```python
from build123d import *

# Parameters (mm, degrees)
SKETCH1_W                                      = 137.49
SKETCH1_H                                      = 96.345
SKETCH1_R                                      = 2.5
SKETCH1_W_2                                    = 10.25
SKETCH1_H_2                                    = 3.4925
BOSS_EXTRUDE1_DEPTH                            = 3.175
CUT_EXTRUDE1_START                             = -1
SKETCH1_3_W                                    = 10.25
SKETCH1_3_H                                    = 3.4925
CUT_EXTRUDE1_DEPTH                             = 5.175
M2_5_CLEARANCE_HOLE1_D                         = 2.9
M2_5_CLEARANCE_HOLE1_CSINK_D                   = 2.95
M2_5_CLEARANCE_HOLE1_CSINK_ANGLE               = 100
MIRROR1_START                                  = -1
MIRROR1_AT_THE_SECOND_PLANE_COPY_1_SKETC_W     = 10.25
MIRROR1_AT_THE_SECOND_PLANE_COPY_1_SKETC_H     = 3.4925
MIRROR1_AT_THE_SECOND_PLANE_COPY_1_DEPTH       = 5.175
MIRROR1_AT_THE_SECOND_PLANE_COPY_2_D           = 2.9
MIRROR1_AT_THE_SECOND_PLANE_COPY_2_CSINK_D     = 2.95
MIRROR1_AT_THE_SECOND_PLANE_COPY_2_CSINK_ANGLE = 100
SKETCH4_W                                      = 82.49
SKETCH4_H                                      = 14
CUT_EXTRUDE2_DEPTH                             = 1
CUT_EXTRUDE2_DEPTH_BACK                        = 4.175
FILLET1_R                                      = 1.5
FILLET2_R                                      = 1
M2_5_CLEARANCE_HOLE2_D                         = 2.9


with BuildPart() as part:
    # Sketch1 → Boss-Extrude1 (new body)
    with BuildSketch(Plane(origin=(0, 0, 0), x_dir=(1, 0, 0), z_dir=(0, 1, 0))):
        Rectangle(SKETCH1_W, SKETCH1_H)
        with Locations((-49.57, 44.1725)):
            Circle(SKETCH1_R, mode=Mode.SUBTRACT)
        with Locations((-58.57, 44.1725)):
            Rectangle(SKETCH1_W_2, SKETCH1_H_2, mode=Mode.SUBTRACT)
        with Locations((-58.57, 44.1725)):
            Rectangle(SKETCH1_W_2, SKETCH1_H_2)
        with Locations((-49.57, 44.1725)):
            Circle(SKETCH1_R)
    extrude(amount=BOSS_EXTRUDE1_DEPTH)

    # Sketch1<3> → Cut-Extrude1 (cut)
    with BuildSketch(Plane(origin=(0, 0, 0), x_dir=(1, 0, 0), z_dir=(0, 1, 0)).offset(CUT_EXTRUDE1_START)):
        with Locations((-58.57, 44.1725)):
            Rectangle(SKETCH1_3_W, SKETCH1_3_H)
    cut_extrude1 = extrude(amount=CUT_EXTRUDE1_DEPTH, mode=Mode.SUBTRACT)

    # M2.5 Clearance Hole1 (through all)
    with Locations(Plane(origin=(0, 3.175, 0), x_dir=(1, 0, 0), z_dir=(0, 1, 0))):
        with Locations((-49.57, 44.1725)):
            m2_5_clearance_hole1 = CounterSinkHole(M2_5_CLEARANCE_HOLE1_D / 2, M2_5_CLEARANCE_HOLE1_CSINK_D / 2, counter_sink_angle=M2_5_CLEARANCE_HOLE1_CSINK_ANGLE)

    # Mirror1: Cut-Extrude1, M2.5 Clearance Hole1 across plane
    add(cut_extrude1.mirror(Plane(origin=(0, 0, 0), x_dir=(0, 0, 1), z_dir=(1, 0, 0))), mode=Mode.SUBTRACT)
    add(m2_5_clearance_hole1.mirror(Plane(origin=(0, 0, 0), x_dir=(0, 0, 1), z_dir=(1, 0, 0))), mode=Mode.SUBTRACT)

    # Mirror1 at the second plane: M2.5 Clearance Hole1, Cut-Extrude1 across plane
    add(m2_5_clearance_hole1.mirror(Plane.XY), mode=Mode.SUBTRACT)
    add(cut_extrude1.mirror(Plane.XY), mode=Mode.SUBTRACT)

    # Mirror1 at the second plane copy 1 sketc → Mirror1 at the second plane copy 1 (cut)
    with BuildSketch(Plane(origin=(0, 0, 0), x_dir=(-1, 0, 0), z_dir=(0, 1, 0)).offset(MIRROR1_START)):
        with Locations((-58.57, 44.1725)):
            Rectangle(MIRROR1_AT_THE_SECOND_PLANE_COPY_1_SKETC_W, MIRROR1_AT_THE_SECOND_PLANE_COPY_1_SKETC_H)
    extrude(amount=MIRROR1_AT_THE_SECOND_PLANE_COPY_1_DEPTH, mode=Mode.SUBTRACT)

    # Mirror1 at the second plane copy 2 (through all)
    with Locations(Plane(origin=(0, 3.175, 0), x_dir=(-1, 0, 0), z_dir=(0, 1, 0))):
        with Locations((-49.57, 44.1725)):
            CounterSinkHole(MIRROR1_AT_THE_SECOND_PLANE_COPY_2_D / 2, MIRROR1_AT_THE_SECOND_PLANE_COPY_2_CSINK_D / 2, counter_sink_angle=MIRROR1_AT_THE_SECOND_PLANE_COPY_2_CSINK_ANGLE)

    # Sketch4 → Cut-Extrude2 (cut, two sides)
    with BuildSketch(Plane(origin=(0, 3.175, 0), x_dir=(1, 0, 0), z_dir=(0, 1, 0))) as cut_extrude2_sk:
        with Locations((19.5, 30.1725)):
            Rectangle(SKETCH4_W, SKETCH4_H)
    extrude(amount=CUT_EXTRUDE2_DEPTH, mode=Mode.SUBTRACT)
    extrude(cut_extrude2_sk.sketch, amount=-CUT_EXTRUDE2_DEPTH_BACK, mode=Mode.SUBTRACT)

    # Fillet1
    fillet1_edges = [part.edges().sort_by_distance(p)[0] for p in [
        (-21.745, 1.5875, -23.1725),
        (-21.745, 1.5875, -37.1725),
        (60.745, 1.5875, -37.1725),
        (60.745, 1.5875, -23.1725),
    ]]
    fillet(fillet1_edges, radius=FILLET1_R)

    # Fillet2
    fillet2_edges = [part.edges().sort_by_distance(p)[0] for p in [
        (-68.745, 1.5875, 48.1725),
        (-68.745, 1.5875, -48.1725),
        (68.745, 1.5875, -48.1725),
        (68.745, 1.5875, 48.1725),
    ]]
    fillet(fillet2_edges, radius=FILLET2_R)

    # M2.5 Clearance Hole2 (through all)
    with Locations(Plane(origin=(0, 3.175, 0), x_dir=(1, 0, 0), z_dir=(0, 1, 0))):
        with Locations((58.745, 15), (58.745, -15)):
            Hole(M2_5_CLEARANCE_HOLE2_D / 2)


solid = part.part
```
Verification items for the finished model (mm, model axes). Round coordinates to 2 decimals unless told otherwise and drop trailing zeros. Order: outer loops, then holes, each group sorted by start corner. A loop starts at its lowest first (then second) coordinate and runs counter-clockwise, first axis right, second up.
1) Cross-section at D-D, the plane x = -10. Record the cut outline in (y, z) (1 decimal).
Geometry says:
outline: (0, -48.2) - (3.2, -48.2) - (3.2, -37.2) - (0, -37.2) - close; (0, -23.2) - (3.2, -23.2) - (3.2, 48.2) - (0, 48.2) - close
2) Cross-section at B-B, the plane z = -15. Record the cut outline in (x, y) (3 decimals), plus the area to 3 significant figures.
Geometry says:
outline: (-68.745, 0) - (57.295, 0) - (57.295, 3.175) - (-68.745, 3.175) - close; (60.195, 0) - (68.745, 0) - (68.745, 3.175) - (60.195, 3.175) - close
area: 427 mm2
3) Material ranges on line 1 (Z direction, x = 49.5, y = 3); line 2 (Z direction, x = 59, y = 2.15); line 3 (Z direction, x = -49.57, y = 2.3), recorded low to high.
Geometry says:
line 1: z = -48.17 to -45.62, -42.72 to -37.17, -23.17 to 42.72, 45.62 to 48.17
line 2: z = -48.17 to -45.92, -42.43 to -37.17, -23.17 to -16.43, -13.57 to 13.57, 16.43 to 42.43, 45.92 to 48.17
line 3: z = -48.17 to -45.62, -42.72 to 42.72, 45.62 to 48.17
4) Cross-section at A-A, the plane x = -55.5. Record the cut outline in (y, z) (1 decimal), plus the area to 3 significant figures.
Geometry says:
outline: (0, -48.2) - (3.2, -48.2) - (3.2, -45.9) - (0, -45.9) - close; (0, -42.4) - (3.2, -42.4) - (3.2, 42.4) - (0, 42.4) - close; (0, 45.9) - (3.2, 45.9) - (3.2, 48.2) - (0, 48.2) - close
area: 284 mm2
5) Draft check along Z on faces 1 (the flat face through (-1, 0, -1)), 2 (the flat face through (60.745, 2, -30)). Enter one of: +Z half, -Z half, draft (parallel to the pull), parting line (faces both ways), or undercut.
Geometry says:
face 1: draft
face 2: undercut
6) Cross-section at C-C, the plane x = 49.57. Give the number of separate pieces and of enclosed holes in the cut face, plus the area to 3 significant figures.
Geometry says:
separate pieces: 4
enclosed holes: 0
area: 243 mm2
